Check sheet for the modelled part. Datum: model origin and axes. Units: mm. Round coordinates to 2 decimals unless told otherwise and drop trailing zeros. Write each loop counter-clockwise with the first axis right and the second up, starting at its lowest first coordinate (ties: lowest second). Pieces come first, ordered by that corner, then holes. Notation, with made-up numbers: M 83.25,46 L 129.25,46 A10 cw 129.25,52 Z; hole C -19,-27 d5. An arc over 180 degrees is marked long. Answer in a Markdown table with one row per item.
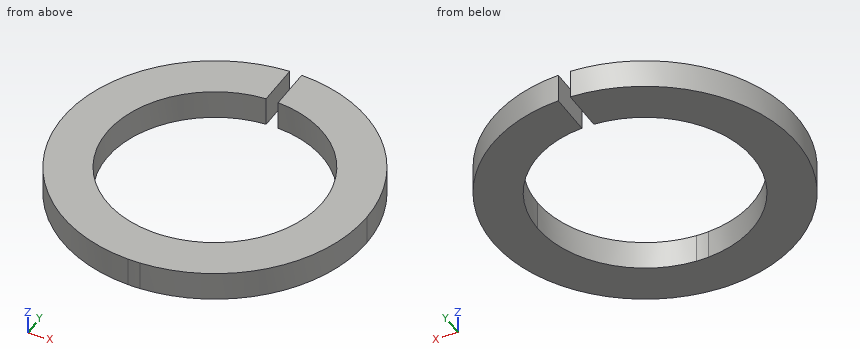
```python
from build123d import *

# Parameters (mm, degrees)
F1_DEPTH = 1.524


# Not quite as in the source:
# - a feature names something its author has since deleted; it is built from what else it names


with BuildPart() as f1:
    # F0 (on Top) → F1 (new body)
    with BuildSketch(Plane.XY):
        with BuildLine():
            ThreePointArc((0.3175, 5.7061737399), (4.1518512437, 3.9272581084), (5.715, 0))
            ThreePointArc((5.715, 0), (4.1518512437, -3.9272581084), (0.3175, -5.7061737399))
            Line((0.3175, -5.7061737399), (0.3175, -8.0582475762))
            ThreePointArc((0.3175, -8.0582475762), (5.8136322123, -5.5890822816), (8.0645, 0))
            ThreePointArc((8.0645, 0), (5.8136322123, 5.5890822816), (0.3175, 8.0582475762))
            Line((0.3175, 8.0582475762), (0.3175, 5.7061737399))
        make_face()
        with BuildLine():
            Line((0.3175, -8.0582475762), (0.3175, -5.7061737399))
            ThreePointArc((0.3175, -5.7061737399), (0, -5.715), (-0.3175, -5.7061737399))
            Line((-0.3175, -5.7061737399), (-0.3175, -8.0582475762))
            ThreePointArc((-0.3175, -8.0582475762), (0, -8.0645), (0.3175, -8.0582475762))
        make_face()
        with BuildLine():
            ThreePointArc((-0.3175, -5.7061737399), (-5.715, 0), (-0.3175, 5.7061737399))
            Line((-0.3175, 5.7061737399), (-0.3175, 8.0582475762))
            ThreePointArc((-0.3175, 8.0582475762), (-8.0645, 0), (-0.3175, -8.0582475762))
            Line((-0.3175, -8.0582475762), (-0.3175, -5.7061737399))
        make_face()
    extrude(amount=F1_DEPTH)


solid = f1.part
```
1. Scan lines: L1, parallel to X at y = -0.75, z = 0.55; L2, parallel to Y at x = -0.5, z = 0.4; L3, parallel to Y at x = 3.25, z = 1.45. Record each from-to range of solid material in increasing order.
Found:
| item | result |
|---|---|
| L1 | x = -8.03 to -5.67, 5.67 to 8.03 |
| L2 | y = -8.05 to -5.69, 5.69 to 8.05 |
| L3 | y = -7.38 to -4.7, 4.7 to 7.38 |
2. Section check B-B, the plane z = 0.2. Record the cut outline in (x, y) (1 decimal).
Found:
| item | result |
|---|---|
| outline | M -0.3,5.7 L -0.3,8.1 A8.1 ccw long 0.3,8.1 L 0.3,5.7 A5.7 cw long Z |
3. Go/stop test with a flat-tipped pin: pin 1 (0.8 mm diameter, centred on y = 7, z = 0.5, fed in from -X). Record where the tip stops, or that it passes through.
Found:
| item | result |
|---|---|
| pin 1 | stops at x = -4.63 |
4. Section check C-C, the plane x = 5. Record the cut outline in (y, z), and give its area (3 significant figures).
Found:
| item | result |
|---|---|
| outline | M -6.33,0 L -2.77,0 L -2.77,1.52 L -6.33,1.52 Z; M 2.77,0 L 6.33,0 L 6.33,1.52 L 2.77,1.52 Z |
| area | 10.8 mm2 |
5. Section check A-A, the plane x = -4.25. Record the cut outline in (y, z).
Found:
| item | result |
|---|---|
| outline | M -6.85,0 L -3.82,0 L -3.82,1.52 L -6.85,1.52 Z; M 3.82,0 L 6.85,0 L 6.85,1.52 L 3.82,1.52 Z |
6. Section check D-D, the plane x = 0. Record the cut outline in (y, z) (1 decimal), and give its area (3 significant figures).
Found:
| item | result |
|---|---|
| outline | M -8.1,0 L -5.7,0 L -5.7,1.5 L -8.1,1.5 Z |
| area | 3.58 mm2 |
